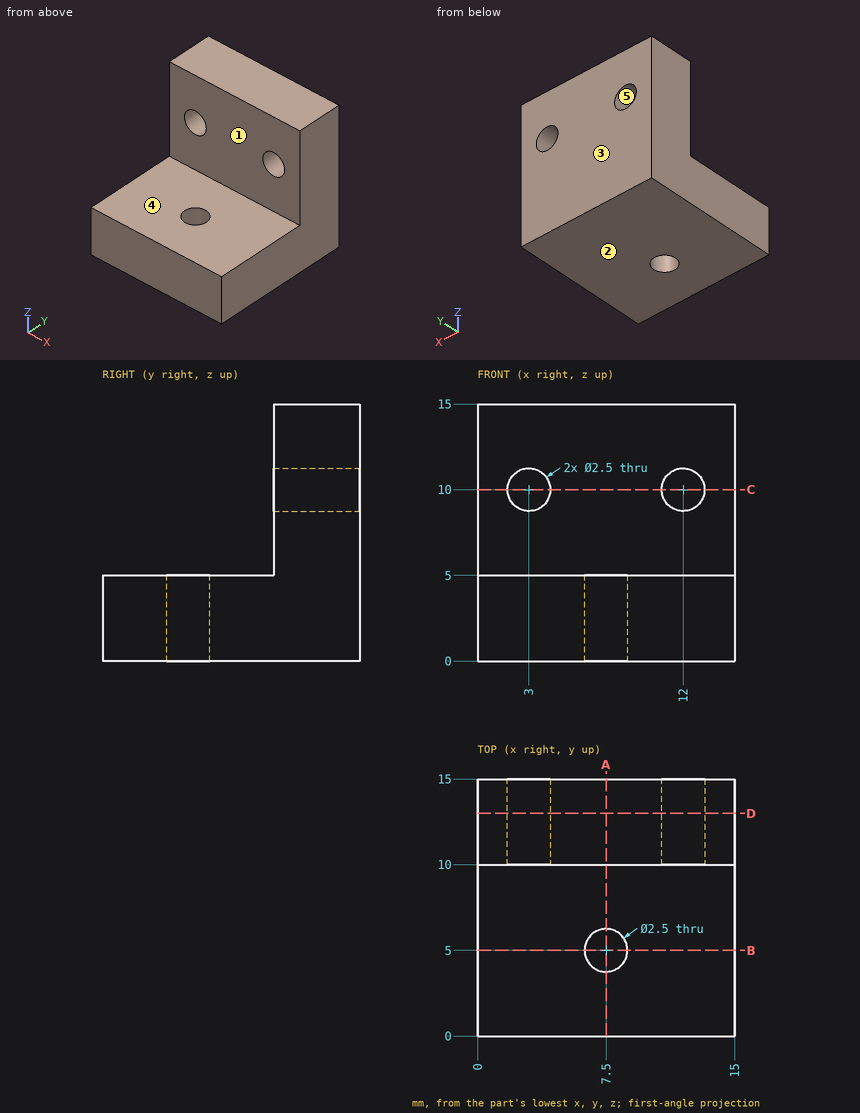
Geometry: see drawing. Coordinates: mm, zero at the bounding-box minimum. A direction names the side the tool comes from. Round coordinates to 2 decimals unless told otherwise and drop trailing zeros. Loops run counter-clockwise (first coordinate to the right, second up) from the corner with the lowest first, then second, coordinate; pieces in that order, holes last. Notation, with made-up numbers: (-2, 86.25) - (10, 86.25) arc R27 ccw to (10, 108.25) - close; hole circle Ø3 at (81, 27.25). An arc over 180 degrees is marked (long way). Use CSV: the item, a comma, the result in double quotes.
Q1. Reachability of the marked faces 1 and 2 from +Z, -Z, +X, -X, +Y, -Y: full face, straight path, thin tool, end or side. Return the list, or none.
Reported:
face 1,"+Z, +X, -X, -Y"
face 2,"-Z, +X, -X, +Y, -Y"
Q2. Ray query, line 1 along X through (y, z) = (13.9, 10); line 2 along Y through (x, z) = (7.5, 3.9); line 3 along Z through (x, y) = (12, 11.8). Return the intervals inside material, ascending.
Reported:
line 1,"0 to 1.75, 4.25 to 10.75, 13.25 to 15"
line 2,"0 to 3.75, 6.25 to 15"
line 3,"0 to 8.75, 11.25 to 15"
Q3. Pin query (flat end, axial travel): pin 1 Ø4 at (x, y) = (7.5, 5) entering from +Z; pin 2 Ø8 at (x, z) = (4.5, 3.5) entering from -Y; pin 3 Ø3 at (x, z) = (12, 10) entering from -Y. Return the tip coordinate at first contact, or that it passes through.
Reported:
pin 1,"z = 5"
pin 2,"y = 0"
pin 3,"y = 10"
Q4. Section query B-B, the plane y = 5. Output: boundary loops of the cut face in (x, z), then the cut area to 3 significant figures.
Reported:
outline,"(0, 0) - (6.25, 0) - (6.25, 5) - (0, 5) - close; (8.75, 0) - (15, 0) - (15, 5) - (8.75, 5) - close"
area,"62.5 mm^2"
Q5. Mould query, pull axis Z, two halves, no side actions, for the marked faces 3, 4 and 5. Classes: pulls with the +Z half, pulls with the -Z half, needs draft (parallel to the pull), parting line crosses it, or undercut.
Reported:
face 3,"needs draft"
face 4,"pulls with the +Z half"
face 5,"undercut"
Q6. Section query A-A, the plane x = 7.5. Output: boundary loops of the cut face in (y, z).
Reported:
outline,"(0, 0) - (3.75, 0) - (3.75, 5) - (0, 5) - close; (6.25, 0) - (15, 0) - (15, 15) - (10, 15) - (10, 5) - (6.25, 5) - close"
Q7. Section query D-D, the plane y = 13. Output: boundary loops of the cut face in (x, z).
Reported:
outline,"(0, 0) - (15, 0) - (15, 15) - (0, 15) - close; hole circle Ø2.5 at (3, 10); hole circle Ø2.5 at (12, 10)"
Q8. Section query C-C, the plane z = 10. Output: boundary loops of the cut face in (x, y).
Reported:
outline,"(0, 10) - (1.75, 10) - (1.75, 15) - (0, 15) - close; (4.25, 10) - (10.75, 10) - (10.75, 15) - (4.25, 15) - close; (13.25, 10) - (15, 10) - (15, 15) - (13.25, 15) - close"
